Read the model definition and answer for the solid it produces. Units are mm, in the model's axes. A direction names the side the tool comes from. Coordinates: 2 decimals unless noted, no trailing zeros. Loops run counter-clockwise (first coordinate to the right, second up) from the corner with the lowest first, then second, coordinate; pieces in that order, holes last.
from build123d import *

# Parameters (mm, degrees)
F1_DEPTH    = 25
F3_R        = 2.54
F4_W        = 50
F4_H        = 30
F5_DEPTH    = 20
F2_W        = 12.7
F2_H        = 25
F6_DEPTH    = 25
F7_T1_DEPTH = 75.655609521
F9_W        = 5
F9_H        = 15
F10_DEPTH   = 10
F11_W       = 7.3
F11_H       = 11.5
F12_DEPTH   = 25.4
F15_R       = 4.9651178244


# Not quite as in the source:
# - a fillet or chamfer that OpenCascade refuses, or shapes differently, is made with other operations: its cross-section is extruded or revolved along the edge and cut away or added
# - a feature names something its author has since deleted; it is built from what else it names


with BuildPart() as f1:
    # F0 (on Top) → F1 (new body)
    with BuildSketch(Plane.XY):
        with BuildLine():
            Line((30, -36.5978047605), (30, 36.5978047605))
            Line((30, 36.5978047605), (-30, 36.5978047605))
            Line((-30, 36.5978047605), (-30, -36.5978047605))
            ThreePointArc((-30, -36.5978047605), (0, -46.4021952395), (30, -36.5978047605))
        make_face()
    extrude(amount=F1_DEPTH)

    # F3
    f3_edges = [f1.edges().sort_by_distance(p)[0] for p in [
        (-30, 36.597805, 12.5),
        (30, 36.597805, 12.5),
    ]]
    fillet(f3_edges, radius=F3_R)

    # F4 (on face) → F5 (cut)
    with BuildSketch(Plane.XY):
        with Locations((0, -31.4021952395)):
            Rectangle(F4_W, F4_H)
    extrude(amount=F5_DEPTH, mode=Mode.SUBTRACT)

    # F2 (on Top) → F6 (cut, through all)
    with BuildSketch(Plane.XY):
        with Locations((0, -33.9021952395)):
            Rectangle(F2_W, F2_H)
    extrude(amount=F6_DEPTH, mode=Mode.SUBTRACT)

    # F7: fillet of radius 1 on 4 edges, made by hand

    # F7_s2 → F7_t1 (cut)
    with BuildSketch(Plane.XZ.offset(-36.5578047605)):
        with BuildLine():
            ThreePointArc((29, 0), (29.7071067812, 0.2928932188), (30, 1))
            Line((30, 1), (30, 0))
            Line((30, 0), (29, 0))
        make_face()
        with BuildLine():
            ThreePointArc((29, 25), (29.7071067812, 24.7071067812), (30, 24))
            Line((30, 24), (30, 25))
            Line((30, 25), (29, 25))
        make_face()
        with BuildLine():
            ThreePointArc((-29, 25), (-29.7071067812, 24.7071067812), (-30, 24))
            Line((-30, 24), (-30, 25))
            Line((-30, 25), (-29, 25))
        make_face()
        with BuildLine():
            ThreePointArc((-29, 0), (-29.7071067812, 0.2928932188), (-30, 1))
            Line((-30, 1), (-30, 0))
            Line((-30, 0), (-29, 0))
        make_face()
    extrude(amount=F7_T1_DEPTH, mode=Mode.SUBTRACT)

    # F9 (on face) → F10 (cut)
    with BuildSketch(Plane(origin=(0, 36.5978047605, 0), x_dir=(-1, 0, 0), z_dir=(0, 1, 0))):
        with Locations((-15.5, 12.5)):
            Rectangle(F9_W, F9_H)
        with Locations((15.5, 12.5)):
            Rectangle(F9_W, F9_H)
        with Locations((-5.5, 12.5)):
            Rectangle(F9_W, F9_H)
        with Locations((5.5, 12.5)):
            Rectangle(F9_W, F9_H)
    extrude(amount=-F10_DEPTH, mode=Mode.SUBTRACT)

    # F11 (on face) → F12 (cut)
    with BuildSketch(Plane(origin=(0, 36.5978047605, 0), x_dir=(-1, 0, 0), z_dir=(0, 1, 0))):
        with Locations((23.35, 12.5)):
            Rectangle(F11_W, F11_H)
    extrude(amount=-F12_DEPTH, mode=Mode.SUBTRACT)

    # F16: sweep along a path in F14
    with BuildLine(Plane.XY.offset(12)) as f16_path:
        Line((-13, -16.4021952395), (-13, -28.9021952395))
        ThreePointArc((-13, -28.9021952395), (0, -41.9021952395), (13, -28.9021952395))
        Line((13, -28.9021952395), (13, -16.4021952395))
    # F15 (on face) → F16 (sweep)
    with BuildSketch(Plane.XZ.offset(16.4021952395)):
        with Locations((-12.9998130724, 11.9997570291)):
            Circle(F15_R)
    sweep(path=f16_path.line)


solid = f1.part
Q1. Straight lines are drawn through the part: probe 1 along X at (y, z) = (31.5, 9); probe 2 along X at (y, z) = (-33, 18.75); probe 3 along X at (y, z) = (-30.5, 9). For each, find the intervals that lie inside material, in ascending order.
Findings below:
probe 1: x = -30 to -27, -19.7 to -18, -13 to -8, -3 to 3, 8 to 13, 18 to 30
probe 2: x = -30 to -25, 25 to 30
probe 3: x = -30 to -25, -16.88 to -8.9, 8.9 to 16.88, 25 to 30
Q2. Which of the six approach directions +Z, -Z, +X, -X, +Y, -Y give full straight-line access (tool end or side, diameter ignored) to faces 1 (the face through (0, -21, 20)), 2 (the face through (-15, 26.598, 13)), 3 (the face through (-30, -1, 12))?
Findings below:
face 1: -Y
face 2: +Y
face 3: +Z, -Z, -X, +Y, -Y
Q3. A cutting plane is placed at A-A (y = 12.5). Give the vertices of the cut face in (x, z).
Findings below:
outline: (-30, 1) arc R1 ccw to (-29, 0) - (29, 0) arc R1 ccw to (30, 1) - (30, 24) arc R1 ccw to (29, 25) - (-29, 25) arc R1 ccw to (-30, 24) - close; hole (-27, 6.75) - (-19.7, 6.75) - (-19.7, 18.25) - (-27, 18.25) - close
Q4. Determine the mould class of faces 4 (the face through (6.35, -34, 22)), 5 (the face through (0, 36.598, 12)), 6 (the face through (30, -2, 12)) for opening direction X: +X half, -X half, draft (parallel to the pull), parting line (faces both ways), or undercut.
Findings below:
face 4: undercut
face 5: draft
face 6: +X half
Q5. A cutting plane is placed at D-D (y = 30). Give the vertices of the cut face in (x, z), then the cut area to 3 significant figures.
Findings below:
outline: (-30, 1) arc R1 ccw to (-29, 0) - (29, 0) arc R1 ccw to (30, 1) - (30, 24) arc R1 ccw to (29, 25) - (-29, 25) arc R1 ccw to (-30, 24) - close; hole (-27, 6.75) - (-19.7, 6.75) - (-19.7, 18.25) - (-27, 18.25) - close; hole (-18, 5) - (-13, 5) - (-13, 20) - (-18, 20) - close; hole (-8, 5) - (-3, 5) - (-3, 20) - (-8, 20) - close; hole (3, 5) - (8, 5) - (8, 20) - (3, 20) - close; hole (13, 5) - (18, 5) - (18, 20) - (13, 20) - close
area: 1,120 mm2
Q6. A cutting plane is placed at B-B (z = 22.5). Give the vertices of the cut face in (x, y).
Findings below:
outline: (-30, -36.6) arc R50.8 ccw to (-6.35, -46) - (-6.35, -21.4) - (6.35, -21.4) - (6.35, -46) arc R50.8 ccw to (30, -36.6) - (30, 34.06) arc R2.54 ccw to (27.46, 36.6) - (-27.46, 36.6) arc R2.54 ccw to (-30, 34.06) - close
Q7. A cutting plane is placed at C-C (x = 0). Give the vertices of the cut face in (y, z).
Findings below:
outline: circle Ø9.93 at (-41.9, 12); (-21.4, 20) - (-16.4, 20) - (-16.4, 0) - (36.6, 0) - (36.6, 25) - (-21.4, 25) - close
Q8. Flat-ended cylindrical pins translate along their axes: pin 1 Ø6 at (x, z) = (-7.5, 12) entering from -Y; pin 2 Ø15 at (x, y) = (-12, -29.5) entering from -Z; pin 3 Ø1.5 at (x, z) = (15, 10) entering from +Y. Find the tip coordinate at first contact, or state that the pin passes through.
Findings below:
pin 1: stops at y = -46.29
pin 2: stops at z = 7.03
pin 3: stops at y = 26.6
